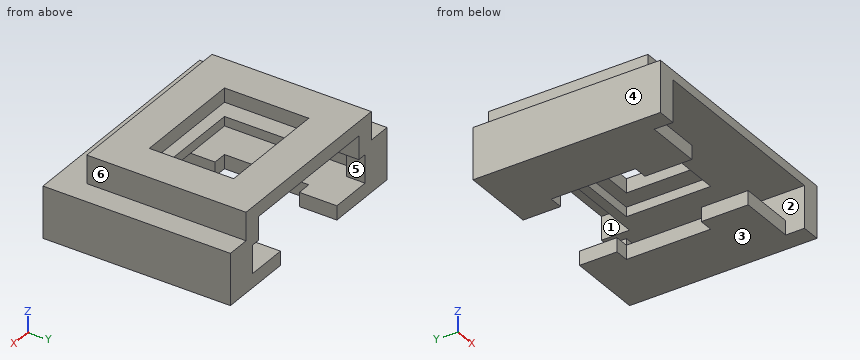
from build123d import *

# Parameters (mm, degrees)
RESSALTO_EXTRUS_O1_DEPTH  = 1.5
RESSALTO_EXTRUS_O2_DEPTH  = 3
ESBO_O2_W                 = 1
ESBO_O2_H                 = 15
ESBO_O2_H_2               = 2
RESSALTO_EXTRUS_O3_DEPTH  = 1
ESBO_O2_4_W               = 1
ESBO_O2_4_H               = 2
ESBO_O2_4_H_2             = 15
RESSALTO_EXTRUS_O4_DEPTH  = 2.5
ESBO_O3_W                 = 20
ESBO_O3_H                 = 17
RESSALTO_EXTRUS_O5_DEPTH  = 1.5
CORTE_EXTRUS_O1_START     = -2
CORTE_EXTRUS_O1_OUTLINE_W = 12
CORTE_EXTRUS_O1_OUTLINE_H = 1.5
CORTE_EXTRUS_O1_DEPTH     = 2
ESBO_O5_W                 = 9
ESBO_O5_H                 = 2
ESBO_O5_H_2               = 16
CORTE_EXTRUS_O2_DEPTH     = 2.5
ESBO_O6_W                 = 12
ESBO_O6_H                 = 9
CORTE_EXTRUS_O3_DEPTH     = 9.5


# Read off the part's stored shape, not the designer's step: Corte-extrusão1
with BuildPart() as part:
    # Esboço1 → Ressalto-extrusão1 (new body)
    with BuildSketch(Plane.XY):
        Polygon((12.5, 10), (-12.5, 10), (-12.5, -10), (-10.5, -10), (-10.5, -8), (10.5, -8), (10.5, -10), (12.5, -10), align=None)
    extrude(amount=-RESSALTO_EXTRUS_O1_DEPTH)

    # Esboço1<3> → Ressalto-extrusão2 (add)
    with BuildSketch(Plane.XY):
        Polygon((-10.5, 8), (-9, 8), (-9, 10), (-12.5, 10), (-12.5, -10), (-10.5, -10), (-10.5, -8), align=None)
        Polygon((9, 10), (9, 8), (10.5, 8), (10.5, -8), (10.5, -10), (12.5, -10), (12.5, 10), align=None)
    extrude(amount=RESSALTO_EXTRUS_O2_DEPTH)

    # Esboço2 → Ressalto-extrusão3 (add)
    with BuildSketch(Plane.XY.offset(3)):
        Polygon((-10, 10), (-12.5, 10), (-12.5, -10), (-10.5, -10), (-10.5, 8), (-10, 8), align=None)
        Polygon((-10.5, 8), (-10.5, -10), (12.5, -10), (12.5, 10), (10, 10), (10, 8), (10, -7), (9, -7), (0, -7), (-9, -7), (-10, -7), (-10, 8), align=None)
        with Locations((-9.5, 0.5)):
            Rectangle(ESBO_O2_W, ESBO_O2_H)
        with Locations((-9.5, 9)):
            Rectangle(ESBO_O2_W, ESBO_O2_H_2)
        Polygon((-8, 8), (-9, 8), (-9, -7), (0, -7), (9, -7), (9, 8), (8, 8), (8, 7), (8, -5), (0, -5), (-8, -5), (-8, 7), align=None)
        with Locations((-8.5, 9)):
            Rectangle(ESBO_O2_W, ESBO_O2_H_2)
        with Locations((8.5, 9)):
            Rectangle(ESBO_O2_W, ESBO_O2_H_2)
        with Locations((9.5, 9)):
            Rectangle(ESBO_O2_W, ESBO_O2_H_2)
        with Locations((9.5, 0.5)):
            Rectangle(ESBO_O2_W, ESBO_O2_H)
        Polygon((8, -5), (8, 7), (0, 7), (0, 0), (0, -5), align=None)
        Polygon((0, 7), (-8, 7), (-8, -5), (0, -5), (0, 0), align=None)
    extrude(amount=RESSALTO_EXTRUS_O3_DEPTH)

    # Esboço2<4> → Ressalto-extrusão4 (add)
    with BuildSketch(Plane.XY.offset(3)):
        with Locations((-8.5, 9)):
            Rectangle(ESBO_O2_4_W, ESBO_O2_4_H)
        with Locations((-9.5, 9)):
            Rectangle(ESBO_O2_4_W, ESBO_O2_4_H)
        with Locations((-9.5, 0.5)):
            Rectangle(ESBO_O2_4_W, ESBO_O2_4_H_2)
        Polygon((-8, 8), (-9, 8), (-9, -7), (0, -7), (9, -7), (9, 8), (8, 8), (8, 7), (8, -5), (0, -5), (-8, -5), (-8, 7), align=None)
        with Locations((9.5, 0.5)):
            Rectangle(ESBO_O2_4_W, ESBO_O2_4_H_2)
        with Locations((8.5, 9)):
            Rectangle(ESBO_O2_4_W, ESBO_O2_4_H)
        with Locations((9.5, 9)):
            Rectangle(ESBO_O2_4_W, ESBO_O2_4_H)
    extrude(amount=RESSALTO_EXTRUS_O4_DEPTH)

    # Esboço3 → Ressalto-extrusão5 (add)
    with BuildSketch(Plane.XY.offset(5.5)):
        with Locations((0, 1.5)):
            Rectangle(ESBO_O3_W, ESBO_O3_H)
    extrude(amount=RESSALTO_EXTRUS_O5_DEPTH)

    # Corte-extrusão1 outline → Corte-extrusão1 (cut)
    with BuildSketch(Plane.XZ.offset(7).offset(CORTE_EXTRUS_O1_START)):
        with Locations((0, 4.75)):
            Rectangle(CORTE_EXTRUS_O1_OUTLINE_W, CORTE_EXTRUS_O1_OUTLINE_H)
    extrude(amount=CORTE_EXTRUS_O1_DEPTH, mode=Mode.SUBTRACT)

    # Esboço5 → Corte-extrusão2 (cut)
    with BuildSketch(Plane(origin=(0, 0, -1.5), x_dir=(-1, 0, 0), z_dir=(0, 0, -1))):
        with Locations((0, 9)):
            Rectangle(ESBO_O5_W, ESBO_O5_H)
        Rectangle(ESBO_O5_W, ESBO_O5_H_2)
    extrude(amount=-CORTE_EXTRUS_O2_DEPTH, mode=Mode.SUBTRACT)

    # Esboço6 → Corte-extrusão3 (cut)
    with BuildSketch(Plane.XY.offset(7)):
        with Locations((0, 1.5)):
            Rectangle(ESBO_O6_W, ESBO_O6_H)
    extrude(amount=-CORTE_EXTRUS_O3_DEPTH, mode=Mode.SUBTRACT)


solid = part.part
Could you check a few things on this model? Use its own coordinates, in mm. Face numbers are marked on the shaded views. A direction names the side the tool comes from. Give positions to 0.01 mm unless a question says otherwise; leave off trailing zeros. Order: outer loops, then holes, each group sorted by start corner. A loop starts at its lowest first (then second) coordinate and runs counter-clockwise, first axis right, second up. Notation, with made-up numbers: M 15.25,31 L 50.25,31 A31 cw 50.25,69 Z; hole C -12.75,25.25 d5. An arc over 180 degrees is marked long. One line per question, with ' | ' between items.
1. We'd pull the mould along X, two halves only. Please class the marked faces 4, 5 and 6: +X half, -X half, draft (parallel to the pull), parting line (faces both ways), or undercut.
Results:
face 4: -X half | face 5: undercut | face 6: +X half
2. I'm going to push flat-ended pins straight in: pin 1 (1.6 mm diameter, centred on x = -7, z = -1, fed in from -Y); pin 2 (0.8 mm diameter, centred on x = -10, z = 1.5, fed in from -Y). Where does each tip first touch, or does it pass through?
Results:
pin 1: y = -8 | pin 2: y = 8
3. If I drill on line 1 (Z direction, x = 6.75, y = -3.25); line 2 (Z direction, x = -10.25, y = 1.25); line 3 (X direction, y = 6, z = 4.25), over which ranges is the centre line in solid material (lowest first)?
Results:
line 1: -1.5 to 0, 3 to 4, 5.5 to 7 | line 2: -1.5 to 0, 3 to 4 | line 3: -10 to -8, 8 to 10
4. I want a section at C-C (x = -3.5). List the corners of the cut face in (y, z) for me, and give its area (3 significant figures).
Results:
outline: M -10,3 L -3,3 L -3,4 L -10,4 Z; M -7,5.5 L -3,5.5 L -3,7 L -7,7 Z; M 6,3 L 7,3 L 7,4 L 6,4 Z; M 6,5.5 L 10,5.5 L 10,7 L 6,7 Z | area: 20.0 mm²
5. I want a section at A-A (z = -1). List the corners of the cut face in (x, y) for me.
Results:
outline: M -12.5,-10 L -10.5,-10 L -10.5,-8 L -4.5,-8 L -4.5,-3 L -6,-3 L -6,6 L -4.5,6 L -4.5,10 L -12.5,10 Z; M 4.5,-8 L 10.5,-8 L 10.5,-10 L 12.5,-10 L 12.5,10 L 4.5,10 L 4.5,6 L 6,6 L 6,-3 L 4.5,-3 Z
6. I want a section at B-B (y = -4.25). List the corners of the cut face in (x, z) for me, and give its area (3 significant figures).
Results:
outline: M -12.5,-1.5 L -4.5,-1.5 L -4.5,0 L -10.5,0 L -10.5,3 L 10.5,3 L 10.5,0 L 4.5,0 L 4.5,-1.5 L 12.5,-1.5 L 12.5,4 L 10,4 L 10,7 L -10,7 L -10,4 L -12.5,4 Z; hole M -8,4 L 8,4 L 8,5.5 L -8,5.5 Z | area: 97.0 mm²
7. I want a section at D-D (z = 6.25). List the corners of the cut face in (x, y) for me.
Results:
outline: M -10,-7 L 10,-7 L 10,10 L -10,10 Z; hole M -6,-3 L 6,-3 L 6,6 L -6,6 Z
8. For the marked faces 1, 2 and 3, which set-ups out of +Z, -Z, +X, -X, +Y, -Y let a thin tool reach every point of the face, with its end or its side?
Results:
face 1: +Y | face 2: -Y | face 3: -Z, +X, -X, +Y, -Y
